Can you work these out from the model? Positions are in its coordinate system, mm. A direction names the side the tool comes from. Coordinates: 2 decimals unless noted, no trailing zeros. Write each loop counter-clockwise with the first axis right and the second up, starting at its lowest first coordinate (ties: lowest second). Pieces come first, ordered by that corner, then holes. Notation, with made-up numbers: (22, 7.5) -> (72, 7.5) arc R11 cw to (72, 19.5) -> close; hole circle Ø4 at (71, 82). An arc over 180 degrees is marked (long way). Use one line per item in the form item = value.
```python
from build123d import *

# Parameters (mm, degrees)
SKETCH_1_W          = 25
SKETCH_1_H          = 8.033880903
EXTRUDE_1_DEPTH     = 3
SKETCH_2_W          = 3
SKETCH_2_H          = 8.033880903
EXTRUDE_2_DEPTH     = 22
SKETCH_3_R          = 3.5
CUT_EXTRUDE_1_DEPTH = 3
SKETCH_4_W          = 15
SKETCH_4_H          = 4.5
CUT_EXTRUDE_2_DEPTH = 2
SKETCH_5_R          = 2.25
CUT_EXTRUDE_3_DEPTH = 2
SKETCH_6_R          = 3.5
CUT_EXTRUDE_4_DEPTH = 3
SKETCH_7_W          = 4.5
SKETCH_7_H          = 15
CUT_EXTRUDE_5_DEPTH = 2
SKETCH_8_R          = 2.25
CUT_EXTRUDE_6_DEPTH = 2


with BuildPart() as part:
    # 草图1 → 凸台-拉伸1 (new body)
    with BuildSketch(Plane(origin=(0, 0, 0), x_dir=(1, 0, 0), z_dir=(0, 1, 0))):
        with Locations((12.5, -4.016940452)):
            Rectangle(SKETCH_1_W, SKETCH_1_H)
    extrude(amount=EXTRUDE_1_DEPTH)

    # 草图2 → 凸台-拉伸2 (add)
    with BuildSketch(Plane(origin=(0, 3, 0), x_dir=(1, 0, 0), z_dir=(0, 1, 0))):
        with Locations((23.5, -4.016940452)):
            Rectangle(SKETCH_2_W, SKETCH_2_H)
    extrude(amount=EXTRUDE_2_DEPTH)

    # 草图3 → 切除-拉伸1 (cut)
    with BuildSketch(Plane(origin=(0, 3, 0), x_dir=(1, 0, 0), z_dir=(0, 1, 0))):
        with Locations(Location((11, -4.033880903, 0), (0, 0, 270))):
            Circle(SKETCH_3_R)
    extrude(amount=-CUT_EXTRUDE_1_DEPTH, mode=Mode.SUBTRACT)

    # 草图4 → 切除-拉伸2 (cut)
    with BuildSketch(Plane(origin=(0, 3, 0), x_dir=(1, 0, 0), z_dir=(0, 1, 0))):
        with Locations((11, -4.033880903)):
            Rectangle(SKETCH_4_W, SKETCH_4_H)
    extrude(amount=-CUT_EXTRUDE_2_DEPTH, mode=Mode.SUBTRACT)

    # 草图5 → 切除-拉伸3 (cut)
    with BuildSketch(Plane(origin=(0, 3, 0), x_dir=(1, 0, 0), z_dir=(0, 1, 0))):
        with Locations((18.5, -4.033880903)):
            Circle(SKETCH_5_R)
        with Locations((3.5, -4.033880903)):
            Circle(SKETCH_5_R)
    extrude(amount=-CUT_EXTRUDE_3_DEPTH, mode=Mode.SUBTRACT)

    # 草图6 → 切除-拉伸4 (cut)
    with BuildSketch(Plane(origin=(25, 0, 0), x_dir=(0, 0, -1), z_dir=(1, 0, 0))):
        with Locations((-4.033880903, 14)):
            Circle(SKETCH_6_R)
    extrude(amount=-CUT_EXTRUDE_4_DEPTH, mode=Mode.SUBTRACT)

    # 草图7 → 切除-拉伸5 (cut)
    with BuildSketch(Plane(origin=(25, 0, 0), x_dir=(0, 0, -1), z_dir=(1, 0, 0))):
        with Locations((-4.033880903, 14)):
            Rectangle(SKETCH_7_W, SKETCH_7_H)
    extrude(amount=-CUT_EXTRUDE_5_DEPTH, mode=Mode.SUBTRACT)

    # 草图8 → 切除-拉伸6 (cut)
    with BuildSketch(Plane(origin=(25, 0, 0), x_dir=(0, 0, -1), z_dir=(1, 0, 0))):
        with Locations((-4.033880903, 6.5)):
            Circle(SKETCH_8_R)
        with Locations((-4.033880903, 21.5)):
            Circle(SKETCH_8_R)
    extrude(amount=-CUT_EXTRUDE_6_DEPTH, mode=Mode.SUBTRACT)


solid = part.part
```
Q1. If I drill on line 1 (Z direction, x = 11, y = 0.75); line 2 (Y direction, x = 4.5, z = 7); line 3 (X direction, y = 6, z = 5.75), over which ranges is the centre line in solid material (lowest first)? Write a range as from..to.
Return value:
line_1 = 0..0.53, 7.53..8.03
line_2 = 0..3
line_3 = 22..23
Q2. Suppose I cut it at A-A (x = 11). Write out the boundary of the cut face in (y, z), then the cut area to 3 significant figures.
Return value:
outline = (0, 0) -> (3, 0) -> (3, 0.53) -> (0, 0.53) -> close; (0, 7.53) -> (3, 7.53) -> (3, 8.03) -> (0, 8.03) -> close
area = 3.10 mm2
Q3. Suppose I cut it at D-D (y = 7.25). Write out the boundary of the cut face in (x, z), then the cut area to 3 significant figures.
Return value:
outline = (22, 0) -> (25, 0) -> (25, 1.78) -> (23, 1.78) -> (23, 6.28) -> (25, 6.28) -> (25, 8.03) -> (22, 8.03) -> close
area = 15.1 mm2
Q4. Thinking about a two-plate mould opening in X: for faces 1 (the flat face through (16, 2, 1.784)), 2 (the flat face through (23, 8, 4)), 3 (the flat face through (15, 0, 4)), 4 (the cylindrical face through (20.75, 2.01, 4.08)), which applies, released by +X, released by -X, zero draft, split by the parting line, or undercut?
Return value:
face_1 = undercut
face_2 = released by +X
face_3 = zero draft
face_4 = undercut
Q5. Will these pins go through, and if not, where does the flat tip stop? pin 1 (2.5 mm diameter, centred on y = 17.5, z = 2.5, fed in from -X); pin 2 (2.5 mm diameter, centred on y = 21, z = 4, fed in from +X); pin 3 (1.4 mm diameter, centred on x = 16.5, z = 5, fed in from +Y).
Return value:
pin_1 = 22
pin_2 = 23
pin_3 = 1
Q6. Suppose I cut it at C-C (z = 4.5). Write out the boundary of the cut face in (x, y).
Return value:
outline = (0, 0) -> (7.53, 0) -> (7.53, 1) -> (1.3, 1) -> (1.3, 3) -> (0, 3) -> close; (14.47, 0) -> (25, 0) -> (25, 4.3) -> (23, 4.3) -> (23, 10.53) -> (22, 10.53) -> (22, 3) -> (20.7, 3) -> (20.7, 1) -> (14.47, 1) -> close; (22, 17.47) -> (23, 17.47) -> (23, 23.7) -> (25, 23.7) -> (25, 25) -> (22, 25) -> close
Q7. For faces 5 (the cylindrical face through (24.01, 4.25, 4.08)), 6 (the flat face through (8, 3, 1)), 7 (the flat face through (5, 1, 4)), 8 (the flat face through (23, 25, 4)), 9 (the flat face through (17, 2, 8.034)), which set-ups out of +Z, -Z, +X, -X, +Y, -Y let a thin tool reach every point of the face, with its end or its side?
Return value:
face_5 = +X
face_6 = +Z, -Z, -X, +Y
face_7 = +Y
face_8 = +Z, -Z, +X, -X, +Y
face_9 = +Z, +X, -X, +Y, -Y
Q8. Suppose I cut it at B-B (y = 17). Write out the boundary of the cut face in (x, z), then the cut area to 3 significant figures.
Return value:
outline = (22, 0) -> (25, 0) -> (25, 1.78) -> (23, 1.78) -> (23, 2.23) -> (22, 2.23) -> close; (22, 5.84) -> (23, 5.84) -> (23, 6.28) -> (25, 6.28) -> (25, 8.03) -> (22, 8.03) -> close
area = 11.5 mm2
